```python
from build123d import *

# Parameters (mm, degrees)
SKETCH_1_R      = 5.25
EXTRUDE_1_DEPTH = 10
SKETCH_2_R      = 18
EXTRUDE_2_DEPTH = 180


with BuildPart() as part:
    # 草图1 → 凸台-拉伸1 (new body)
    with BuildSketch(Plane.XY):
        with BuildLine():
            Line((21, 0), (21, -48.626933041))
            Line((21, -48.626933041), (63.112159322, -24.313466521))
            ThreePointArc((63.112159322, -24.313466521), (91.798692801, -32), (84.112159322, -60.686533479))
            Line((84.112159322, -60.686533479), (42, -85))
            Line((42, -85), (84.112159322, -109.313466521))
            ThreePointArc((84.112159322, -109.313466521), (91.798692801, -138), (63.112159322, -145.686533479))
            Line((63.112159322, -145.686533479), (21, -121.373066959))
            Line((21, -121.373066959), (21, -170))
            ThreePointArc((21, -170), (0, -191), (-21, -170))
            Line((-21, -170), (-21, -121.373066959))
            Line((-21, -121.373066959), (-63.112159322, -145.686533479))
            ThreePointArc((-63.112159322, -145.686533479), (-91.798692801, -138), (-84.112159322, -109.313466521))
            Line((-84.112159322, -109.313466521), (-42, -85))
            Line((-42, -85), (-84.112159322, -60.686533479))
            ThreePointArc((-84.112159322, -60.686533479), (-91.798692801, -32), (-63.112159322, -24.313466521))
            Line((-63.112159322, -24.313466521), (-21, -48.626933041))
            Line((-21, -48.626933041), (-21, 0))
            ThreePointArc((-21, 0), (0, 21), (21, 0))
        make_face()
        with Locations((0, -10)):
            Circle(SKETCH_1_R, mode=Mode.SUBTRACT)
        with Locations((64.951905284, -47.5)):
            Circle(SKETCH_1_R, mode=Mode.SUBTRACT)
        with Locations((64.951905284, -122.5)):
            Circle(SKETCH_1_R, mode=Mode.SUBTRACT)
        with Locations((0, -160)):
            Circle(SKETCH_1_R, mode=Mode.SUBTRACT)
        with Locations((-64.951905284, -122.5)):
            Circle(SKETCH_1_R, mode=Mode.SUBTRACT)
        with Locations((-64.951905284, -47.5)):
            Circle(SKETCH_1_R, mode=Mode.SUBTRACT)
    extrude(amount=EXTRUDE_1_DEPTH)

    # 草图2 → 凸台-拉伸2 (add)
    with BuildSketch(Plane(origin=(0, 0, 0), x_dir=(-1, 0, 0), z_dir=(0, 0, -1))):
        with Locations(Location((0, -85.20347481, 0), (0, 0, 180))):
            Circle(SKETCH_2_R)
    extrude(amount=EXTRUDE_2_DEPTH)


solid = part.part
```
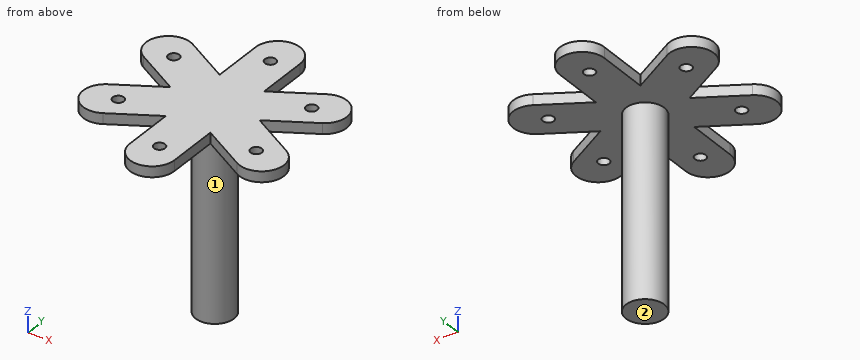
Part model, mm, in its own coordinate system. Face numbers are marked on the shaded views. A direction names the side the tool comes from. Give positions to 0.01 mm unless a question says otherwise; leave off trailing zeros. Write each loop counter-clockwise with the first axis right and the second up, starting at its lowest first coordinate (ties: lowest second). Pieces come first, ordered by that corner, then holes. Notation, with made-up numbers: (-14.75, 66.5) -> (10.25, 66.5) arc R29 cw to (10.25, 100.5) -> close; hole circle Ø7 at (54.5, 80). An arc over 180 degrees is marked (long way). Put each result on its own line as item: value. Start each with the question number.
Item 1: Cut at A-A (y = -160). List the corners of the cut face in (x, z), then the cut area to 3 significant figures.
Item 2: Cut at D-D (z = -43). List the corners of the cut face in (x, y).
Item 3: Wall check: L1, parallel to Y at x = 0, z = 5; L2, parallel to Z at x = 67.5, y = -128.5; L3, parallel to Y at x = 6.5, z = -97. Give the ranges that are in metal, low to high. Write a range as [from, to].
Item 4: Cut at C-C (y = -92.5). List the corners of the cut face in (x, z).
Item 5: Cut at B-B (x = 0). List the corners of the cut face in (y, z).
Item 6: Pin check, flat tips, straight feed: pin 1 Ø5 at (y, z) = (-17.5, 5.5) entering from -X; pin 2 Ø8 at (y, z) = (-16.5, 4) entering from +X; pin 3 Ø13.5 at (x, y) = (64.95, -47.5) entering from -Z. Stop position of each tip, or through.
Item 7: Which spindle directions (+Z, -Z, +X, -X, +Y, -Y) get a long thin tool onto all of the face, cutting with end or side? Do the marked faces 1 and 2. Say none if no direction does.
Answer list:
1. outline: (-21, 0) -> (-5.25, 0) -> (-5.25, 10) -> (-21, 10) -> close; (5.25, 0) -> (21, 0) -> (21, 10) -> (5.25, 10) -> close
1. area: 315 mm2
2. outline: circle Ø36 at (0, -85.2)
3. L1: y = [-191, -165.25], [-154.75, -15.25], [-4.75, 21]
3. L2: z = [0, 10]
3. L3: y = [-101.99, -68.42]
4. outline: (-54.99, 0) -> (-16.45, 0) -> (-16.45, -180) -> (16.45, -180) -> (16.45, 0) -> (54.99, 0) -> (54.99, 10) -> (-54.99, 10) -> close
5. outline: (-191, 0) -> (-165.25, 0) -> (-165.25, 10) -> (-191, 10) -> close; (-154.75, 0) -> (-103.2, 0) -> (-103.2, -180) -> (-67.2, -180) -> (-67.2, 0) -> (-15.25, 0) -> (-15.25, 10) -> (-154.75, 10) -> close; (-4.75, 0) -> (21, 0) -> (21, 10) -> (-4.75, 10) -> close
6. pin 1: stops at x = -21
6. pin 2: stops at x = 21
6. pin 3: stops at z = 0
7. face 1: -Z
7. face 2: -Z, +X, -X, +Y, -Y
